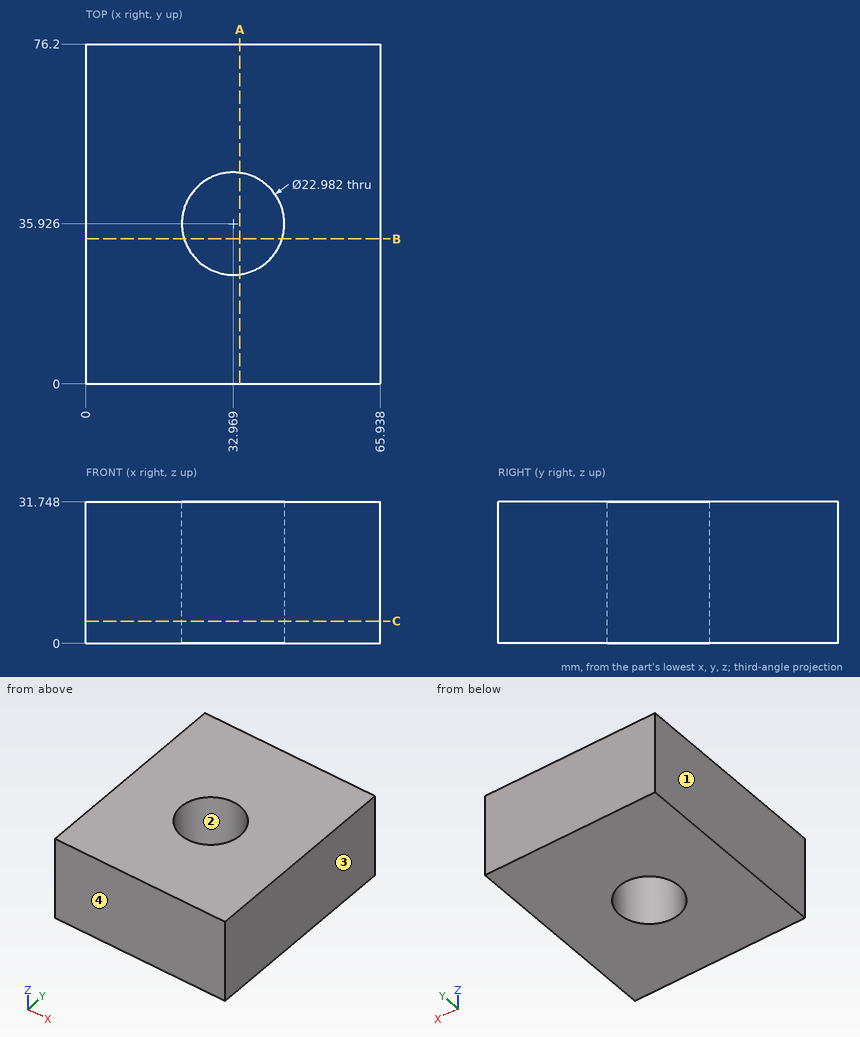
The drawing under review shows one solid part. Ordinate dimensions are in mm from its lowest x, y, z. Round coordinates to 2 decimals unless told otherwise and drop trailing zeros. Loops run counter-clockwise (first coordinate to the right, second up) from the corner with the lowest first, then second, coordinate; pieces in that order, holes last. Notation, with made-up numbers: (-13, -30) -> (34, -30) arc R19 cw to (34, -4) -> close; hole circle Ø6 at (-17, 25). An arc over 180 degrees is marked (long way). Answer in a Markdown table with one row per item.
1) Consider section C-C, the plane z = 5. Write out the cut boundary in (x, y).
Taken from the geometry:
| item | result |
|---|---|
| outline | (0, 0) -> (65.94, 0) -> (65.94, 76.2) -> (0, 76.2) -> close; hole circle Ø22.98 at (32.97, 35.93) |
2) Consider section B-B, the plane y = 32.5. Write out the cut boundary in (x, z).
Taken from the geometry:
| item | result |
|---|---|
| outline | (0, 0) -> (22, 0) -> (22, 31.75) -> (0, 31.75) -> close; (43.94, 0) -> (65.94, 0) -> (65.94, 31.75) -> (43.94, 31.75) -> close |
3) Consider section A-A, the plane x = 34.5. Write out the cut boundary in (y, z) (1 decimal), plus the area to 3 significant figures.
Taken from the geometry:
| item | result |
|---|---|
| outline | (0, 0) -> (24.5, 0) -> (24.5, 31.7) -> (0, 31.7) -> close; (47.3, 0) -> (76.2, 0) -> (76.2, 31.7) -> (47.3, 31.7) -> close |
| area | 1,700 mm² |
4) For pin 1 Ø1 at (x, y) = (24.5, 32) entering from +Z, flat-tipped, find the tip position at first contact; note if it passes through.
Taken from the geometry:
| item | result |
|---|---|
| pin 1 | passes through |
5) Wall thickness on line 1 along X through (y, z) = (36.5, 19.5) (1 decimal); line 2 along Y through (x, z) = (41, 30) (1 decimal); line 3 along Y through (x, z) = (37, 5) (1 decimal): over which ranges is each line inside the solid? List them lowest first.
Taken from the geometry:
| item | result |
|---|---|
| line 1 | x = 0 to 21.5, 44.4 to 65.9 |
| line 2 | y = 0 to 27.7, 44.1 to 76.2 |
| line 3 | y = 0 to 25.2, 46.7 to 76.2 |
6) Draft analysis for pull direction X (two halves, no side actions). For the marked faces 1, 2, 3 and 4, state which applies: pulls with the +X half, pulls with the -X half, needs draft (parallel to the pull), parting line crosses it, or undercut.
Taken from the geometry:
| item | result |
|---|---|
| face 1 | pulls with the -X half |
| face 2 | undercut |
| face 3 | pulls with the +X half |
| face 4 | needs draft |
